The model under review builds one solid part; all positions refer to its coordinate system, in mm. Face numbers are marked on the shaded views. A direction names the side the tool comes from. Give positions to 0.01 mm unless a question says otherwise; leave off trailing zeros. Loops run counter-clockwise (first coordinate to the right, second up) from the corner with the lowest first, then second, coordinate; pieces in that order, holes last. Notation, with made-up numbers: M 12.5,16.25 L 34.5,16.25 A20 ccw 34.5,32.25 Z; hole C 75,1.25 d8. An arc over 180 degrees is marked long. Return JSON: item names as keys, results as strings. Group by question number.
```python
from build123d import *

# Parameters (mm, degrees)
SKETCH1_W           = 50.8
SKETCH1_H           = 25.4
BOSS_EXTRUDE1_DEPTH = 50.8
SKETCH2_W           = 19.05
SKETCH2_H           = 19.05
CUT_EXTRUDE1_DEPTH  = 50.8
SKETCH3_R           = 6.35
BOSS_EXTRUDE2_DEPTH = 6.35


with BuildPart() as part:
    # Sketch1 → Boss-Extrude1 (new body)
    with BuildSketch(Plane.XY):
        with Locations((25.4, 12.7)):
            Rectangle(SKETCH1_W, SKETCH1_H)
    extrude(amount=BOSS_EXTRUDE1_DEPTH)

    # Sketch2 → Cut-Extrude1 (cut)
    with BuildSketch(Plane.XY.offset(50.8)):
        with Locations((25.4, 9.525)):
            Rectangle(SKETCH2_W, SKETCH2_H)
    extrude(amount=-CUT_EXTRUDE1_DEPTH, mode=Mode.SUBTRACT)

    # Sketch3 → Boss-Extrude2 (add)
    with BuildSketch(Plane(origin=(0, 25.4, 0), x_dir=(1, 0, 0), z_dir=(0, 1, 0))):
        with Locations(Location((25.4, -25.4, 0), (0, 0, 270))):
            Circle(SKETCH3_R)
    extrude(amount=BOSS_EXTRUDE2_DEPTH)


solid = part.part
```
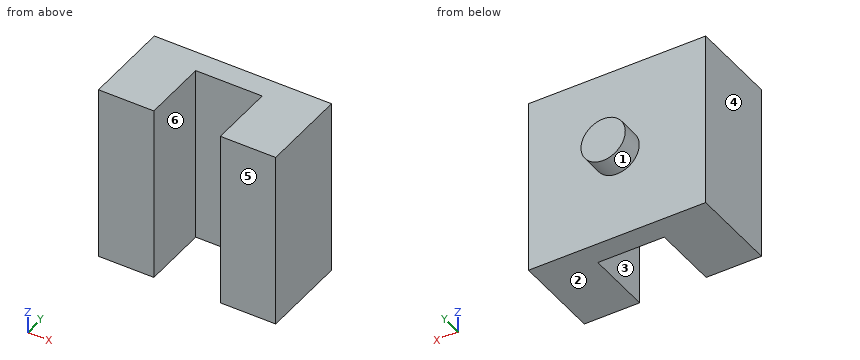
(1) Add section A-A (y = 8). Write out the cut boundary in (x, z) (3 decimals), and give its area (3 significant figures).
(2) Add section C-C (z = 25.4). Write out the cut boundary in (x, y) (3 decimals), and give its area (3 significant figures).
(3) Add section B-B (x = 25.4). Write out the cut boundary in (y, z).
(4) For the marked faces 1, 2 and 3, list the 3-axis set-ups (+Z, -Z, +X, -X, +Y, -Y) from which the entire face can be reached by the end or side of a thin tool; tool diameter is ignored.
(5) Mouldability with a two-part tool opening along X and no side actions: class the marked faces 4, 5 and 6 as released by +X, released by -X, zero draft, split by the parting line, or undercut.
(6) For probe 1 along X at (y, z) = (15.5, 30) (3 decimals); probe 2 along Y at (x, z) = (19, 48); probe 3 along Y at (x, z) = (41, 9), list the stretches that pass through material, from the lowest coordinate up.
(7) Add section D-D (y = 26.5). Write out the cut boundary in (x, z).
(8) For pin 1 (10 mm diameter, centred on x = 21, z = 10.5, fed in from -Y), flat-tipped, find the tip position at first contact; note if it passes through.
Verdict:
{
 "1": {"outline": "M 0,0 L 15.875,0 L 15.875,50.8 L 0,50.8 Z; M 34.925,0 L 50.8,0 L 50.8,50.8 L 34.925,50.8 Z", "area": "1,610 mm²"},
 "2": {"outline": "M 0,0 L 15.875,0 L 15.875,19.05 L 34.925,19.05 L 34.925,0 L 50.8,0 L 50.8,25.4 L 31.75,25.4 L 31.75,31.75 L 19.05,31.75 L 19.05,25.4 L 0,25.4 Z", "area": "1,010 mm²"},
 "3": {"outline": "M 19.05,0 L 25.4,0 L 25.4,19.05 L 31.75,19.05 L 31.75,31.75 L 25.4,31.75 L 25.4,50.8 L 19.05,50.8 Z"},
 "4": {"face 1": "+Y", "face 2": "-Z, +X, -X, +Y, -Y", "face 3": "+Z, -Z, -Y"},
 "5": {"face 4": "released by -X", "face 5": "zero draft", "face 6": "undercut"},
 "6": {"probe 1": "x = 0 to 15.875, 34.925 to 50.8", "probe 2": "y = 19.05 to 25.4", "probe 3": "y = 0 to 25.4"},
 "7": {"outline": "C 25.4,25.4 d12.7"},
 "8": {"pin 1": "stops at y = 19.05"}
}
